Read the model definition and answer for the solid it produces. Units are mm, in the model's axes. A direction names the side the tool comes from. Give positions to 0.01 mm unless a question says otherwise; leave off trailing zeros. Order: outer loops, then holes, each group sorted by start corner. A loop starts at its lowest first (then second) coordinate and runs counter-clockwise, first axis right, second up. Notation, with made-up numbers: (-25.75, 40) -> (22.25, 40) arc R25 ccw to (22.25, 60) -> close; hole circle Ø1 at (19, 77.25). An arc over 180 degrees is marked (long way). Use one line per item in the form item = value.
```python
from build123d import *

# Parameters (mm, degrees)
SKETCH4_R           = 11.2395
CUT_EXTRUDE1_DEPTH  = 9.525
SKETCH5_W           = 2.921
SKETCH5_H           = 2.921
BOSS_EXTRUDE1_DEPTH = 1.8415


with BuildPart() as part:
    # Sketch3 → Revolve2 (revolve)
    with BuildSketch(Plane(origin=(0, 0, 0), x_dir=(0, 0, -1), z_dir=(1, 0, 0)), mode=Mode.PRIVATE) as revolve2_sk:
        with BuildLine():
            Line((0, 0), (38.1, 0))
            ThreePointArc((38.1, 0), (40.889807909, 6.735192091), (47.625, 9.525))
            Line((47.625, 9.525), (57.15, 9.525))
            Line((57.15, 9.525), (57.15, 12.7))
            Line((57.15, 12.7), (38.1, 12.7))
            ThreePointArc((38.1, 12.7), (18.1414881, 9.65411308), (0, 0.79375))
            Line((0, 0.79375), (0, 0))
        make_face()
    revolve(revolve2_sk.sketch.rotate(Axis((0, 0, 0), (0, 0, -1)), 90), axis=Axis((0, 0, 0), (0, 0, -1)))

    # Sketch4 → Cut-Extrude1 (cut)
    with BuildSketch(Plane(origin=(0, 0, -57.15), x_dir=(-1, 0, 0), z_dir=(0, 0, -1))):
        Circle(SKETCH4_R)
    extrude(amount=-CUT_EXTRUDE1_DEPTH, mode=Mode.SUBTRACT)

    # Sketch5 → Boss-Extrude1 (add)
    with BuildSketch(Plane(origin=(0, 11.43, 0), x_dir=(1, 0, 0), z_dir=(0, 1, 0))):
        with Locations((0, 55.6895)):
            Rectangle(SKETCH5_W, SKETCH5_H)
    boss_extrude1 = extrude(amount=-BOSS_EXTRUDE1_DEPTH)

    # Mirror1: Boss-Extrude1 across plane
    add(boss_extrude1.mirror(Plane.ZX))


solid = part.part
```
Item 1: The part is cut by section A-A on z = -53. Give the vertices of the cut face in (x, y), and give its area (3 significant figures).
Checks:
outline = circle Ø25.4 at (0, 0); hole circle Ø22.48 at (0, 0)
area = 110 mm²
Item 2: Given pin 1 Ø4 at (x, y) = (0, -7) entering from +Z; pin 2 Ø1.5 at (x, y) = (3.5, -3.5) entering from -Z; pin 3 Ø2 at (x, y) = (-1.5, 2.5) entering from +Z, each flat-ended and moving along its own axis, determine where each tip first touches the part or whether it passes through.
Checks:
pin_1 = -6.94
pin_2 = -39.99
pin_3 = -1.67
Item 3: Straight lines are drawn through the part: L1, parallel to Y at x = 0, z = -54.75; L2, parallel to Y at x = 0, z = -50.75; L3, parallel to Y at x = -1, z = -17. For each, find the intervals that lie inside material, in ascending order. Write a range as from..to.
Checks:
L1 = -12.7..-9.59, 9.59..12.7
L2 = -12.7..-11.24, 11.24..12.7
L3 = -9.23..9.23
Item 4: Determine the mould class of faces 1 (the flat face through (-1.46, -10, -56)), 2 (the flat face through (0, -10, -54.229)), 3 (the flat face through (0, 0, 0)) for opening direction Z: +Z half, -Z half, draft (parallel to the pull), parting line (faces both ways), or undercut.
Checks:
face_1 = draft
face_2 = undercut
face_3 = +Z half
Item 5: Which of the six approach directions +Z, -Z, +X, -X, +Y, -Y give full straight-line access (tool end or side, diameter ignored) to faces 4 (the flat face through (0, 9.588, -56)), 5 (the flat face through (0, 10, -54.229)), 6 (the cylindrical face through (-10.1, 7.7, -47.5))?
Checks:
face_4 = -Z
face_5 = none
face_6 = +Z, -Z
